Source: CAD feature listing. Evaluate the final solid. Frame: model axes, mm. Give positions to 0.01 mm unless a question says otherwise; leave off trailing zeros. Loops run counter-clockwise (first coordinate to the right, second up) from the corner with the lowest first, then second, coordinate; pieces in that order, holes last. Notation, with made-up numbers: (-18, 8.5) - (38, 8.5) arc R26 cw to (38, 47.5) - close; hole circle Ø2 at (-11, 22.5). An arc over 180 degrees is marked (long way). Put each result on its own line as item: value.
Autodesk Inventor part; units mm, degrees
ref_plane "YZ Plane" through (0, 0, 0) normal (1, 0, 0) x (0, 1, 0)
ref_plane "XZ Plane" through (0, 0, 0) normal (0, 1, 0) x (-1, 0, 0)
ref_plane "XY Plane" through (0, 0, 0) normal (0, 0, 1) x (1, 0, 0)
sketch "草图2" plane through (0, 0, 0) normal (0, 1, 0) x (-1, 0, 0)
  line L0 (-21, 21) -> (21, 21)
  line L1 (21, 21) -> (21, -21)
  line L2 (21, -21) -> (-21, -21)
  line L3 (-21, -21) -> (-21, 21)
  line L4 (-21, 21) -> (21, -21) construction
  line L5 (21, 21) -> (-21, -21) construction
  point P0 (0, 0)
  dimension "d3" = 42
  dimension "d4" = 42
extrude "拉伸2" add sketch "草图2" along normal blind 3
sketch "草图7" plane through (0, 0, 0) normal (0, -1, 0) x (1, 0, 0)
  circle A0 centre (0, 0) radius 11.5
  circle A1 centre (-15.5, 15.5) radius 1.75
  circle A2 centre (-15.5, -15.5) radius 1.75
  circle A3 centre (15.5, -15.5) radius 1.75
  circle A4 centre (15.5, 15.5) radius 1.75
  dimension "d17" = 23
  dimension "d18" = 3.5
  dimension "d19" = 15.5
  dimension "d20" = 15.5
  dimension "d21" = 15.5
  dimension "d22" = 15.5
extrude "拉伸6" cut sketch "草图7" against normal blind 3
sketch "草图14" plane through (-21, 0, 21) normal (0, 0, 1) x (1, 0, 0)
  line L0 (42, 0) -> (0, 0)
  line L1 (42, 0) -> (42, 3)
  line L2 (0, 3) -> (42, 3)
  line L3 (0, 0) -> (0, 3)
  point P0 (21, 0)
extrude "拉伸13" add sketch "草图14" along normal blind 20
sketch "草图15" plane through (0, 0, 0) normal (0, -1, 0) x (1, 0, 0)
  line L0 (0, 53.4) -> (0, -33.4) construction
  circle A0 centre (10, 33) radius 3
  line L1 (-21, 41) -> (21, 41)
  circle A1 centre (-10, 33) radius 3
  point P0 (0, 0)
  dimension "d51" = 6
  dimension "d52" = 10
  dimension "d53" = 8
extrude "拉伸15" cut sketch "草图15" against normal blind 10
properties part number "电机座3"
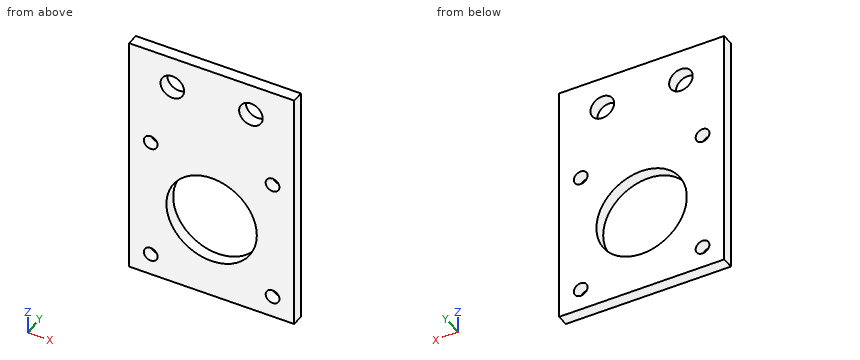
1) Section query A-A, the plane z = 33. Output: boundary loops of the cut face in (x, y), plus the area to 3 significant figures.
Check result:
outline: (-21, 0) - (-13, 0) - (-13, 3) - (-21, 3) - close; (-7, 0) - (7, 0) - (7, 3) - (-7, 3) - close; (13, 0) - (21, 0) - (21, 3) - (13, 3) - close
area: 90.0 mm²
2) Material intervals for line 1 along Z through (x, y) = (-15.5, 0.8); line 2 along Z through (x, y) = (10, 0.6); line 3 along Z through (x, y) = (0, 0.65), sorted ascending. Write a range as [from, to].
Check result:
line 1: [-21, -17.25], [-13.75, 13.75], [17.25, 41]
line 2: [-21, -5.68], [5.68, 30], [36, 41]
line 3: [-21, -11.5], [11.5, 41]
3) Section query C-C, the plane y = 1.8. Output: boundary loops of the cut face in (x, z), plus the area to 3 significant figures.
Check result:
outline: (-21, -21) - (21, -21) - (21, 41) - (-21, 41) - close; hole circle Ø3.5 at (-15.5, -15.5); hole circle Ø3.5 at (-15.5, 15.5); hole circle Ø6 at (-10, 33); hole circle Ø23 at (0, 0); hole circle Ø6 at (10, 33); hole circle Ø3.5 at (15.5, -15.5); hole circle Ø3.5 at (15.5, 15.5)
area: 2,090 mm²
4) Section query D-D, the plane z = 10. Output: boundary loops of the cut face in (x, y).
Check result:
outline: (-21, 0) - (-5.68, 0) - (-5.68, 3) - (-21, 3) - close; (5.68, 0) - (21, 0) - (21, 3) - (5.68, 3) - close
5) Section query B-B, the plane x = 0. Output: boundary loops of the cut face in (y, z), plus the area to 3 significant figures.
Check result:
outline: (0, -21) - (3, -21) - (3, -11.5) - (0, -11.5) - close; (0, 11.5) - (3, 11.5) - (3, 41) - (0, 41) - close
area: 117 mm²
6) Pin query (flat end, axial travel): P1, Ø2, axis at x = -15.5, z = -15.5, coming from the +Y side. Return the tip coordinate at first contact, or that it passes through.
Check result:
P1: through
